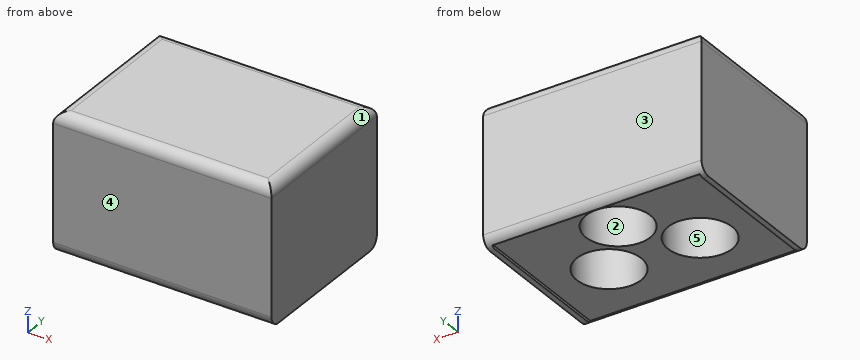
from build123d import *

# Parameters (mm, degrees)
F0_W        = 103.4230701625
F0_H        = 75.2167738974
F1_DEPTH    = 65.024
F2_T        = -2.54
F3_T1_DEPTH = 128.8230701625
F3_T3_DEPTH = 100.6167738974
F4_W        = 31.4045592836
F4_H        = 70.1367738974
F5_DEPTH    = 61.214
F6_R        = 15.24
F7_DEPTH    = 49.022


# Not quite as in the source:
# - a fillet or chamfer that OpenCascade refuses, or shapes differently, is made with other operations: its cross-section is extruded or revolved along the edge and cut away or added


with BuildPart() as f1:
    # F0 (on Top) → F1 (new body)
    with BuildSketch(Plane.XY):
        with Locations((6.9133061916, -6.8211276084)):
            Rectangle(F0_W, F0_H)
    extrude(amount=F1_DEPTH)

    # F2
    f2_openings = [f1.faces().sort_by_distance(p)[0] for p in [
        (6.913306, -6.821128, 0),
    ]]
    offset(amount=F2_T, openings=f2_openings)

    # F3: fillet of radius 5.08 on 6 edges, made by hand

    # F3_s2 → F3_t1 (cut)
    with BuildSketch(Plane.YZ.offset(-57.4982288897)):
        with BuildLine():
            ThreePointArc((-44.4295145571, 59.944), (-42.9416170056, 63.5361024484), (-39.3495145571, 65.024))
            Line((-39.3495145571, 65.024), (-44.4295145571, 65.024))
            Line((-44.4295145571, 65.024), (-44.4295145571, 59.944))
        make_face()
        with BuildLine():
            ThreePointArc((30.7872593403, 59.944), (29.2993617887, 63.5361024484), (25.7072593403, 65.024))
            Line((25.7072593403, 65.024), (30.7872593403, 65.024))
            Line((30.7872593403, 65.024), (30.7872593403, 59.944))
        make_face()
        with BuildLine():
            ThreePointArc((30.7872593403, 5.08), (29.2993617887, 1.4878975516), (25.7072593403, 0))
            Line((25.7072593403, 0), (30.7872593403, 0))
            Line((30.7872593403, 0), (30.7872593403, 5.08))
        make_face()
        with BuildLine():
            ThreePointArc((-44.4295145571, 5.08), (-42.9416170056, 1.4878975516), (-39.3495145571, 0))
            Line((-39.3495145571, 0), (-44.4295145571, 0))
            Line((-44.4295145571, 0), (-44.4295145571, 5.08))
        make_face()
    extrude(amount=F3_T1_DEPTH, mode=Mode.SUBTRACT)

    # F3_s4 → F3_t3 (cut)
    with BuildSketch(Plane.XZ.offset(-43.4872593403)):
        with BuildLine():
            ThreePointArc((-44.7982288897, 59.944), (-43.3103313381, 63.5361024484), (-39.7182288897, 65.024))
            Line((-39.7182288897, 65.024), (-44.7982288897, 65.024))
            Line((-44.7982288897, 65.024), (-44.7982288897, 59.944))
        make_face()
        with BuildLine():
            ThreePointArc((58.6248412728, 59.944), (57.1369437213, 63.5361024484), (53.5448412728, 65.024))
            Line((53.5448412728, 65.024), (58.6248412728, 65.024))
            Line((58.6248412728, 65.024), (58.6248412728, 59.944))
        make_face()
    extrude(amount=F3_T3_DEPTH, mode=Mode.SUBTRACT)

    # F4 (on face) → F5 (join)
    with BuildSketch(Plane(origin=(0, 0, 62.484), x_dir=(1, 0, 0), z_dir=(0, 0, -1))):
        Polygon((24.3728496134, 41.8895145571), (-10.8536696061, 41.8895145571), (-10.8536696061, -28.2472593403), (56.0848412728, -28.2472593403), (56.0848412728, 41.8895145571), align=None)
        with Locations((-26.5559492479, 6.8211276084)):
            Rectangle(F4_W, F4_H)
    extrude(amount=F5_DEPTH)

    # F6 (on face) → F7 (cut)
    with BuildSketch(Plane(origin=(0, 0, 1.27), x_dir=(1, 0, 0), z_dir=(0, 0, -1))):
        with Locations((-15.0351587272, 13.1098517179)):
            Circle(F6_R)
        with Locations((28.1448412728, 13.1098517179)):
            Circle(F6_R)
        with Locations((7.1306948804, -12.0557340983)):
            Circle(F6_R)
    extrude(amount=-F7_DEPTH, mode=Mode.SUBTRACT)


solid = f1.part
Work out the finished part from the listing and answer in its coordinate system (mm). Face numbers are marked on the shaded views. A direction names the side the tool comes from. Coordinates: 2 decimals unless noted, no trailing zeros. Loops run counter-clockwise (first coordinate to the right, second up) from the corner with the lowest first, then second, coordinate; pieces in that order, holes last. Notation, with made-up numbers: M 25,-33.5 L 73,-33.5 A23 ccw 73,-5.5 Z; hole C -34.75,4 d8. An arc over 180 degrees is marked long. Answer in a Markdown table with one row per item. Add a question column.
1. Find section B-B, the plane z = 45. Write down the section's boundary in (x, y), then the cut area to 3 significant figures.
2. The mould has two halves that part along X. Classify the marked faces 1, 2 and 3: pulls with the +X half, pulls with the -X half, needs draft (parallel to the pull), parting line crosses it, or undercut.
3. Find section D-D, the plane x = 28. Write down the section's boundary in (y, z).
4. Find section A-A, the plane x = -18. Write down the section's boundary in (y, z), then the cut area to 3 significant figures.
5. Find section C-C, the plane y = -5.5. Write down the section's boundary in (x, z).
6. Flat-ended cylindrical pins translate along their axes: P1, Ø21, axis at x = -11, y = -12, coming from the -Z side; P2, Ø0.5, axis at x = 18.5, z = 1, coming from the -Y side; P3, Ø8, axis at x = -21, y = 22.5, coming from the -Z side. Find the tip coordinate at first contact, or state that the pin passes through.
7. Consider L1, parallel to X at y = -24, z = 42.5; L2, parallel to Y at x = -6.5, z = 9; L3, parallel to X at y = -4.5, z = 36.5. Determine where each line is inside the solid, lowest interval first.
8. A tool of negligible diameter and unlimited length cuts with its end or side. For the marked faces 4 and 5, from which of +Z, -Z, +X, -X, +Y, -Y can it reach the whole face along a straight path? Write none if from no direction.
Reported:
| question | item | result |
|---|---|---|
| 1 | outline | M -44.8,-44.43 L 58.62,-44.43 L 58.62,30.79 L -44.8,30.79 Z; hole C -15.04,-13.11 d30.48; hole C 7.13,12.06 d30.48; hole C 28.14,-13.11 d30.48 |
| 1 | area | 5,590 mm^2 |
| 2 | face 1 | pulls with the +X half |
| 2 | face 2 | undercut |
| 2 | face 3 | needs draft |
| 3 | outline | M -44.43,5.08 A5.08 ccw -41.89,0.68 L -41.89,1.27 L -28.35,1.27 L -28.35,50.29 L 2.13,50.29 L 2.13,1.27 L 28.25,1.27 L 28.25,0.68 A5.08 ccw 30.79,5.08 L 30.79,59.94 A5.08 ccw 25.71,65.02 L -39.35,65.02 A5.08 ccw -44.43,59.94 Z |
| 4 | outline | M -44.43,5.08 A5.08 ccw -41.89,0.68 L -41.89,1.27 L -28.06,1.27 L -28.06,50.29 L 1.84,50.29 L 1.84,1.27 L 28.25,1.27 L 28.25,0.68 A5.08 ccw 30.79,5.08 L 30.79,59.94 A5.08 ccw 25.71,65.02 L -39.35,65.02 A5.08 ccw -44.43,59.94 Z |
| 4 | area | 3,320 mm^2 |
| 5 | outline | M -44.8,0 L -42.26,0 L -42.26,1.27 L -28.24,1.27 L -28.24,50.29 L -1.83,50.29 L -1.83,1.27 L 14.94,1.27 L 14.94,50.29 L 41.35,50.29 L 41.35,1.27 L 56.08,1.27 L 56.08,0 L 58.62,0 L 58.62,59.94 A5.08 ccw 53.54,65.02 L -39.72,65.02 A5.08 ccw -44.8,59.94 Z |
| 6 | P1 | stops at z = 50.29 |
| 6 | P2 | stops at y = -42.69 |
| 6 | P3 | stops at z = 1.27 |
| 7 | L1 | x = -44.8 to -25.7, -4.37 to 17.48, 38.81 to 58.62 |
| 7 | L2 | y = -44.43 to -25.74, -0.48 to 5.24, 18.87 to 30.79 |
| 7 | L3 | x = -44.8 to -27.61, -2.46 to 15.57, 40.72 to 58.62 |
| 8 | face 4 | +Z, -Z, +X, -X, -Y |
| 8 | face 5 | -Z |
